Build history of the part. All positions in model axes, mm. A direction names the side the tool comes from. Round coordinates to 2 decimals unless told otherwise and drop trailing zeros. Write each loop counter-clockwise with the first axis right and the second up, starting at its lowest first coordinate (ties: lowest second). Pieces come first, ordered by that corner, then holes. Notation, with made-up numbers: M 29.25,23.25 L 41.25,23.25 A8 ccw 41.25,27.25 Z; hole C -15.5,43 d2. An arc over 180 degrees is marked long. Write item = value, one per line.
from build123d import *

# Parameters (mm, degrees)
SKETCH1_W           = 30.988
SKETCH1_H           = 23.3045
BOSS_EXTRUDE1_DEPTH = 3.81
CUT_EXTRUDE1_DEPTH  = 29.718
BOSS_EXTRUDE2_DEPTH = 2.54
SKETCH4_W           = 25.908
SKETCH4_H           = 18.2245
CUT_EXTRUDE2_DEPTH  = 2.54


with BuildPart() as part:
    # Sketch1 → Boss-Extrude1 (new body)
    with BuildSketch(Plane(origin=(0, 0, 0), x_dir=(1, 0, 0), z_dir=(0, 1, 0))):
        with Locations((15.494, 11.65225)):
            Rectangle(SKETCH1_W, SKETCH1_H)
    extrude(amount=BOSS_EXTRUDE1_DEPTH)

    # Sketch2 → Cut-Extrude1 (cut)
    with BuildSketch(Plane(origin=(30.988, 0, 0), x_dir=(0, 0, -1), z_dir=(1, 0, 0))):
        Polygon((6.57225, 0), (9.11225, 2.54), (14.19225, 2.54), (16.73225, 0), align=None)
    extrude(amount=-CUT_EXTRUDE1_DEPTH, mode=Mode.SUBTRACT)

    # Sketch3 → Boss-Extrude2 (add)
    with BuildSketch(Plane.XZ):
        with BuildLine():
            Line((2.54, -0.6604), (28.448, -0.6604))
            ThreePointArc((28.448, -0.6604), (29.0576, -1.27), (28.448, -1.8796))
            Line((28.448, -1.8796), (2.54, -1.8796))
            ThreePointArc((2.54, -1.8796), (1.9304, -1.27), (2.54, -0.6604))
        make_face()
        with BuildLine():
            Line((2.54, -21.4249), (28.448, -21.4249))
            ThreePointArc((28.448, -21.4249), (29.0576, -22.0345), (28.448, -22.6441))
            Line((28.448, -22.6441), (2.54, -22.6441))
            ThreePointArc((2.54, -22.6441), (1.9304, -22.0345), (2.54, -21.4249))
        make_face()
    extrude(amount=BOSS_EXTRUDE2_DEPTH)

    # Sketch4 → Cut-Extrude2 (cut)
    with BuildSketch(Plane.XZ):
        with Locations((15.494, -11.65225)):
            Rectangle(SKETCH4_W, SKETCH4_H)
    extrude(amount=-CUT_EXTRUDE2_DEPTH, mode=Mode.SUBTRACT)


solid = part.part
1. Tool access for faces 5 (the face through (16, -1, -22.644)), 6 (the face through (1.93, -1.25, -22.05)), 7 (the face through (28.448, 1, -5)), 8 (the face through (15, -1, -21.425)), 9 (the face through (1.91, 1.29, -15.44)): list every direction of +Z, -Z, +X, -X, +Y, -Y with a clear straight run to the whole face (end or side of a thin tool).
Responses:
face_5 = -Z, +X, -X, -Y
face_6 = -X, -Y
face_7 = -Y
face_8 = +X, -X, -Y
face_9 = +X, -Y
2. Flat gauge pins, fed straight in: pin 1 (0.8 mm diameter, centred on x = 20.5, y = -2, fed in from -Z); pin 2 (1.3 mm diameter, centred on x = 21, y = -1.5, fed in from +Z); pin 3 (1.5 mm diameter, centred on x = 9.5, z = -15, fed in from -Y). Where does each tip first touch, or does it go through?
Responses:
pin_1 = -22.64
pin_2 = -0.66
pin_3 = 2.54
3. Band-saw the part on D-D (y = 1.25). List the corners of the cut face in (x, z), plus the area to 3 significant figures.
Responses:
outline = M 0,-23.3 L 30.99,-23.3 L 30.99,-15.48 L 28.45,-15.48 L 28.45,-20.76 L 2.54,-20.76 L 2.54,-15.48 L 1.27,-15.48 L 1.27,-7.82 L 2.54,-7.82 L 2.54,-2.54 L 28.45,-2.54 L 28.45,-7.82 L 30.99,-7.82 L 30.99,0 L 0,0 Z
area = 221 mm²
4. Band-saw the part on C-C (z = -1.27). List the corners of the cut face in (x, y).
Responses:
outline = M 0,0 L 1.93,0 L 1.93,-2.54 L 29.06,-2.54 L 29.06,0 L 30.99,0 L 30.99,3.81 L 0,3.81 Z
5. Probe probe 1 along X at (y, z) = (2.25, -19.25); probe 2 along Z at (x, y) = (8, 2); probe 3 along Z at (x, y) = (4, -0.5). List the from-to ranges inside material, lowest first.
Responses:
probe_1 = 0 to 2.54, 28.45 to 30.99
probe_2 = -23.3 to -20.76, -2.54 to 0
probe_3 = -22.64 to -21.42, -1.88 to -0.66
6. Band-saw the part on A-A (y = -1.25). List the corners of the cut face in (x, z), plus the area to 3 significant figures.
Responses:
outline = M 2.54,-22.64 L 28.45,-22.64 A0.61 ccw 28.45,-21.42 L 2.54,-21.42 A0.61 ccw Z; M 2.54,-1.88 L 28.45,-1.88 A0.61 ccw 28.45,-0.66 L 2.54,-0.66 A0.61 ccw Z
area = 65.5 mm²
7. Band-saw the part on B-B (x = 28). List the corners of the cut face in (y, z), plus the area to 3 significant figures.
Responses:
outline = M -2.54,-22.64 L 0,-22.64 L 0,-23.3 L 3.81,-23.3 L 3.81,0 L 0,0 L 0,-0.66 L -2.54,-0.66 L -2.54,-1.88 L 0,-1.88 L 0,-2.54 L 2.54,-2.54 L 2.54,-20.76 L 0,-20.76 L 0,-21.42 L -2.54,-21.42 Z
area = 48.7 mm²
8. Mould opens along Z. For faces 1 (the face through (16, 2.54, -12)), 2 (the face through (16, -2.54, -22)), 3 (the face through (15, -1, -0.66)), 4 (the face through (29.057, -1.252, -22.021)) say: pulls with the +Z half, pulls with the -Z half, needs draft (parallel to the pull), parting line crosses it, or undercut.
Responses:
face_1 = undercut
face_2 = needs draft
face_3 = pulls with the +Z half
face_4 = undercut
